Geometry: see drawing. Coordinates: mm, zero at the bounding-box minimum. A direction names the side the tool comes from. Give positions to 0.01 mm unless a question says otherwise; leave off trailing zeros. Order: outer loops, then holes, each group sorted by start corner. A loop starts at its lowest first (then second) coordinate and runs counter-clockwise, first axis right, second up. Notation, with made-up numbers: M -20,4 L 30,4 A26 ccw 30,23 Z; hole C 3,-6 d9. An arc over 180 degrees is marked long. Answer as a JSON object with one key per item and string values. Group by question number.
1. Set-up query: the marked faces 3 and 4. Return all of +Z, -Z, +X, -X, +Y, -Y with unobstructed straight access to the full face (end or side cutting, diameter ignored); none if empty.
2. Section query B-B (z = 50.8). Output: boundary loops of the cut face in (x, y) (3 decimals).
3. Section query C-C (z = 87). Output: boundary loops of the cut face in (x, y) (3 decimals), plus the area to 3 significant figures.
4. Section query A-A (x = 44.45). Output: boundary loops of the cut face in (y, z) (3 decimals).
5. Material intervals for L1, parallel to Z at x = 63.5, y = 0.7 (3 decimals); L2, parallel to Y at x = 27, z = 44.5 (3 decimals); L3, parallel to X at y = 2.35, z = 12.7 (3 decimals), sorted ascending. Write a range as [from, to].
6. Section query D-D (y = 11.25). Output: boundary loops of the cut face in (x, z) (3 decimals).
7. Pull-direction query (X, two-part tool) for the marked faces 1 and 2; classes: +X half, -X half, draft (parallel to the pull), parting line (faces both ways), or undercut.
8. Pin query (flat end, axial travel): P1, Ø15, axis at x = 44.45, z = 50.8, coming from the -Y side; P2, Ø7.5, axis at x = 63.5, z = 88.9, coming from the +Y side (3 decimals); P3, Ø4, axis at x = 63.5, z = 12.7, coming from the -Y side; P4, Ø5, axis at y = 7, z = 38, coming from the -X side. Return the tip coordinate at first contact, or that it passes through.
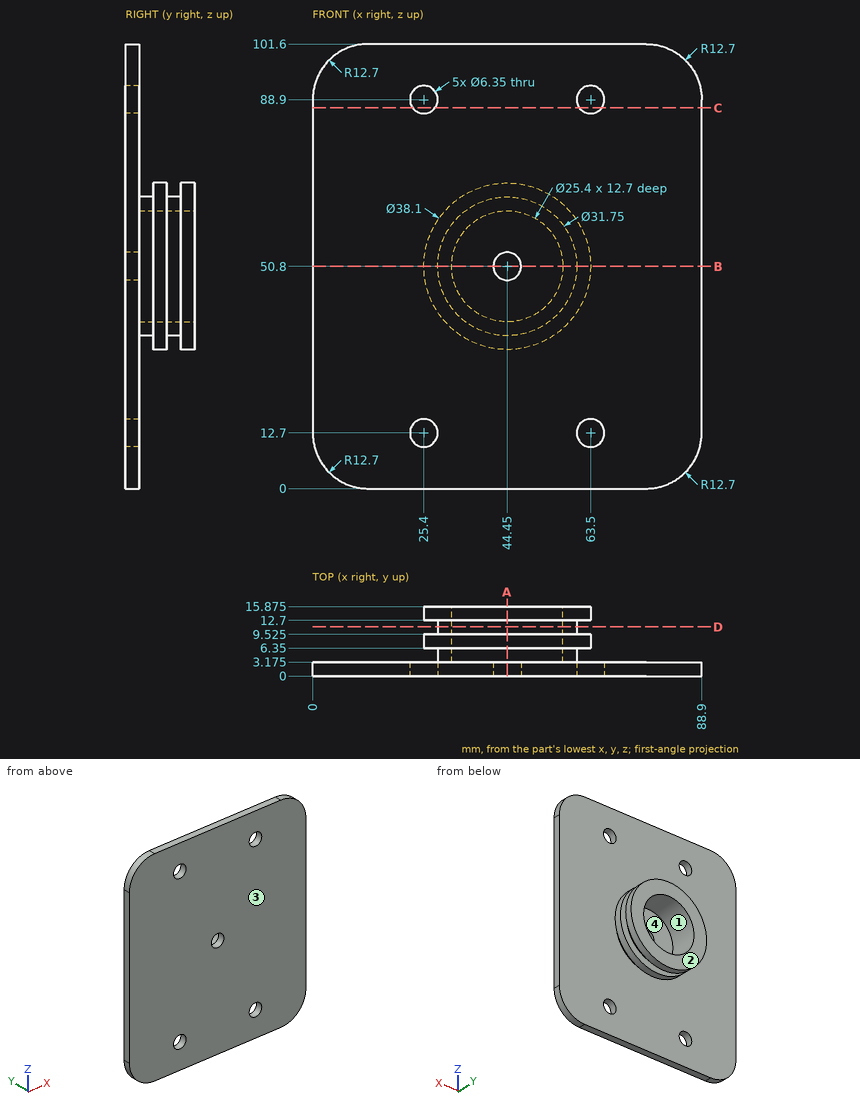
Answer sheet:
{
 "1": {"face 3": "+Z, -Z, +X, -X, -Y", "face 4": "+Y"},
 "2": {"outline": "M 0,0 L 41.275,0 L 41.275,3.175 L 31.75,3.175 L 31.75,15.875 L 25.4,15.875 L 25.4,12.7 L 28.575,12.7 L 28.575,9.525 L 25.4,9.525 L 25.4,6.35 L 28.575,6.35 L 28.575,3.175 L 0,3.175 Z; M 47.625,0 L 88.9,0 L 88.9,3.175 L 60.325,3.175 L 60.325,6.35 L 63.5,6.35 L 63.5,9.525 L 60.325,9.525 L 60.325,12.7 L 63.5,12.7 L 63.5,15.875 L 57.15,15.875 L 57.15,3.175 L 47.625,3.175 Z"},
 "3": {"outline": "M 0,0 L 22.856,0 L 22.856,3.175 L 0,3.175 Z; M 27.944,0 L 60.956,0 L 60.956,3.175 L 27.944,3.175 Z; M 66.044,0 L 88.9,0 L 88.9,3.175 L 66.044,3.175 Z", "area": "250 mm^2"},
 "4": {"outline": "M 0,0 L 3.175,0 L 3.175,34.925 L 6.35,34.925 L 6.35,31.75 L 9.525,31.75 L 9.525,34.925 L 12.7,34.925 L 12.7,31.75 L 15.875,31.75 L 15.875,38.1 L 3.175,38.1 L 3.175,47.625 L 0,47.625 Z; M 0,53.975 L 3.175,53.975 L 3.175,63.5 L 15.875,63.5 L 15.875,69.85 L 12.7,69.85 L 12.7,66.675 L 9.525,66.675 L 9.525,69.85 L 6.35,69.85 L 6.35,66.675 L 3.175,66.675 L 3.175,101.6 L 0,101.6 Z"},
 "5": {"L1": "[0, 9.525], [15.875, 85.725], [92.075, 101.6]", "L2": "[0, 3.175], [6.35, 9.525], [12.7, 15.875]", "L3": "[0, 22.225], [28.575, 60.325], [66.675, 88.9]"},
 "6": {"outline": "C 44.45,50.8 d31.75; hole C 44.45,50.8 d25.4"},
 "7": {"face 1": "undercut", "face 2": "draft"},
 "8": {"P1": "y = 0", "P2": "y = 3.175", "P3": "through", "P4": "x = 28.42"}
}
